Design review of the part built by this model. Coordinates are the model's own, in mm. Give positions to 0.01 mm unless a question says otherwise; leave off trailing zeros. Loops run counter-clockwise (first coordinate to the right, second up) from the corner with the lowest first, then second, coordinate; pieces in that order, holes last.
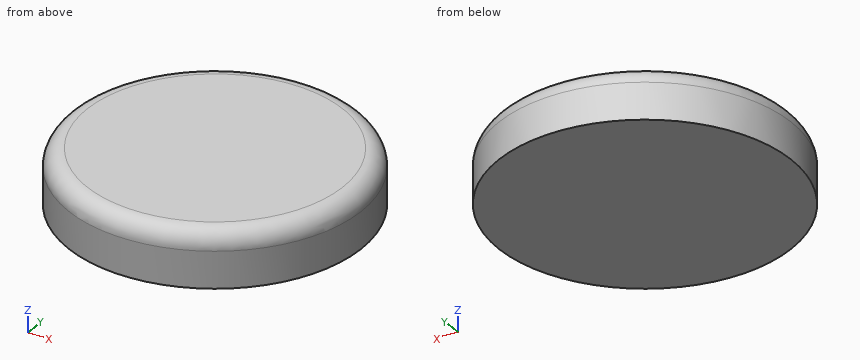
from build123d import *

# Parameters (mm, degrees)
SKETCH1_R           = 40
BOSS_EXTRUDE1_DEPTH = 15
FILLET1_R           = 5
SCALE1_SCALE        = 2


with BuildPart() as part:
    # Sketch1 → Boss-Extrude1 (new body)
    with BuildSketch(Plane.XY):
        Circle(SKETCH1_R)
    extrude(amount=BOSS_EXTRUDE1_DEPTH)

    # Fillet1
    fillet1_edges = [part.edges().sort_by_distance(p)[0] for p in [
        (-40, 0, 15),
    ]]
    fillet(fillet1_edges, radius=FILLET1_R)


with BuildPart() as part_1:
    # Scale1: scaled about (0, 0, 7.387306203)
    add(part.part.scale(SCALE1_SCALE).moved(Location((0, 0, -7.387306203))))


solid = part_1.part
Q1. Take a section at A-A (z = 5.25). Give the boundary of the cut face in (x, y).
Results:
outline: circle Ø160 at (0, 0)
Q2. Insertion check: pin 1 (1.5 mm diameter, centred on x = 40.5, y = -59, fed in from +Z); pin 2 (1.5 mm diameter, centred on y = -16.5, z = 4.5, fed in from -X); pin 3 (8 mm diameter, centred on x = -2, z = -4.5, fed in from -Y). Each pin has a flat end and moves straight along its axis. Give the tip position at first contact, or say it passes through.
Results:
pin 1: stops at z = 22.58
pin 2: stops at x = -78.43
pin 3: stops at y = -80
Q3. Take a section at B-B (z = 19). Give the boundary of the cut face in (x, y), plus the area to 3 significant figures.
Results:
outline: circle Ø155.39 at (0, 0)
area: 19,000 mm2
Q4. Wall thickness on line 1 (Y direction, x = -12.5, z = -2.5); line 2 (X direction, y = -61, z = 3.5); line 3 (Y direction, x = 58, z = 8.75): over which ranges is each line inside the solid? List them lowest first.
Results:
line 1: y = -79.02 to 79.02
line 2: x = -51.76 to 51.76
line 3: y = -55.1 to 55.1
